Can you work these out from the model? Positions are in its coordinate system, mm. Give positions to 0.01 mm unless a question says otherwise; leave off trailing zeros. Write each loop counter-clockwise with the first axis right and the second up, starting at its lowest first coordinate (ties: lowest second). Pieces come first, ordered by that corner, then holes.
Autodesk Inventor part; units mm, degrees
ref_plane "YZ Plane" through (0, 0, 0) normal (1, 0, 0) x (0, 1, 0)
ref_plane "XZ Plane" through (0, 0, 0) normal (0, 1, 0) x (-1, 0, 0)
ref_plane "XY Plane" through (0, 0, 0) normal (0, 0, 1) x (1, 0, 0)
sketch "スケッチ1" plane through (0, 0, 0) normal (0, 1, 0) x (-1, 0, 0)
  circle A0 centre (0, 0) radius 5
  dimension "d0" = 10
extrude "押し出し1" add sketch "スケッチ1" along normal blind 193
sketch "スケッチ2" plane through (0, 193, 0) normal (0, 1, 0) x (1, 0, 0)
  circle A0 centre (0, 0) radius 4
  circle A1 centre (0, 0) radius 5
  dimension "d3" = 8
  dimension "d4" = 10
extrude "押し出し2" cut sketch "スケッチ2" against normal blind 193
sketch "スケッチ3" plane through (0, 193, 0) normal (0, 1, 0) x (1, 0, 0)
  circle A0 centre (0, 0) radius 6
  circle A1 centre (0, 0) radius 4
  dimension "d7" = 12
  dimension "d9" = 8
extrude "押し出し3" add sketch "スケッチ3" against normal blind 193
sketch "スケッチ4" plane through (0, 0, 0) normal (0, -1, 0) x (1, 0, 0)
  circle A0 centre (0, 0) radius 6
  dimension "d12" = 12
extrude "押し出し4" add sketch "スケッチ4" along normal blind 20
properties part number "射出_軸" material "アルミニウム 6061"
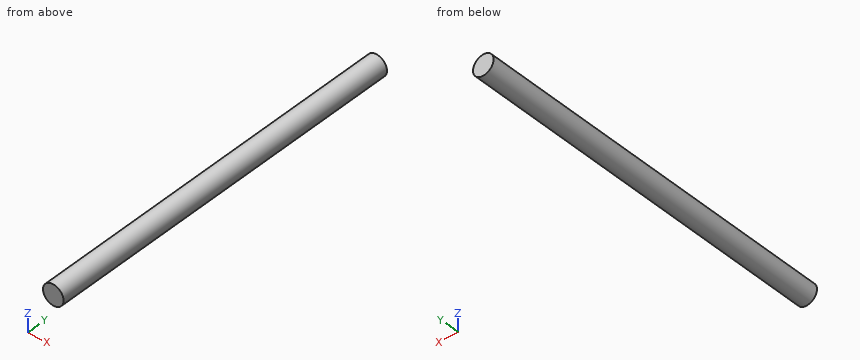
1) Suppose I cut it at B-B on x = 3.75. Write out the boundary of the cut face in (y, z), plus the area to 3 significant figures.
Values follow:
outline: (-20, -4.68) - (193, -4.68) - (193, 4.68) - (-20, 4.68) - close
area: 2,000 mm2
2) Suppose I cut it at A-A on y = 18.5. Write out the boundary of the cut face in (x, z).
Values follow:
outline: circle Ø12 at (0, 0)
3) For pin 1 Ø3 at (y, z) = (60, -4.5) entering from +X; pin 2 Ø5 at (x, y) = (-3.5, 54.5) entering from -Z; pin 3 Ø4 at (y, z) = (157, -3) entering from -X; pin 4 Ø4 at (x, y) = (0.5, 53) entering from -Z, each with a flat end and sliding along its axis, tell me the tip position at first contact or that it passes through.
Values follow:
pin 1: stops at x = 5.2
pin 2: stops at z = -5.92
pin 3: stops at x = -5.92
pin 4: stops at z = -6
4) Please list where these lines run through material, in increasing order: L1, parallel to Z at x = 5, y = 175.5; L2, parallel to Z at x = 4.75, y = 101; L3, parallel to X at y = 113.5, z = -1.
Values follow:
L1: z = -3.32 to 3.32
L2: z = -3.67 to 3.67
L3: x = -5.92 to 5.92
